Study the drawing (mm; zero at the part's minimum x, y, z) and answer. A direction names the side the tool comes from. Give positions to 0.01 mm unless a question says otherwise; leave off trailing zeros. Write each loop counter-clockwise with the first axis right and the second up, starting at its lowest first coordinate (ties: lowest second). Pieces come first, ordered by that corner, then holes.
1) Find section D-D (y = 28). Determine the outline of the cut face in (x, z).
2) Determine the mould class of the marked faces 4, 5, 6 and 7 for opening direction Y: pulls with the +Y half, pulls with the -Y half, needs draft (parallel to the pull), parting line crosses it, or undercut.
3) Straight lines are drawn through the part: probe 1 along X at (y, z) = (113, 23); probe 2 along Z at (x, y) = (17, 113); probe 3 along Y at (x, z) = (12, 19.5). For each, find the intervals that lie inside material, in ascending order.
4) Find section A-A (z = 23). Determine the outline of the cut face in (x, y).
5) Find section B-B (z = 40). Determine the outline of the cut face in (x, y).
6) Given pin 1 Ø18.5 at (x, z) = (20.5, 32.5) entering from -Y; pin 2 Ø1.2 at (x, z) = (28.5, 2.5) entering from +Y; pin 3 Ø4 at (x, z) = (32, 29) entering from +Y, each flat-ended and moving along its own axis, determine where each tip first touches the part or whether it passes through.
7) Find section C-C (x = 17). Determine the outline of the cut face in (y, z).
8) A tool of negligible diameter and unlimited length cuts with its end or side. For the marked faces 1, 2 and 3, from which of +Z, -Z, +X, -X, +Y, -Y can it reach the whole face along a straight path? Write none if from no direction.
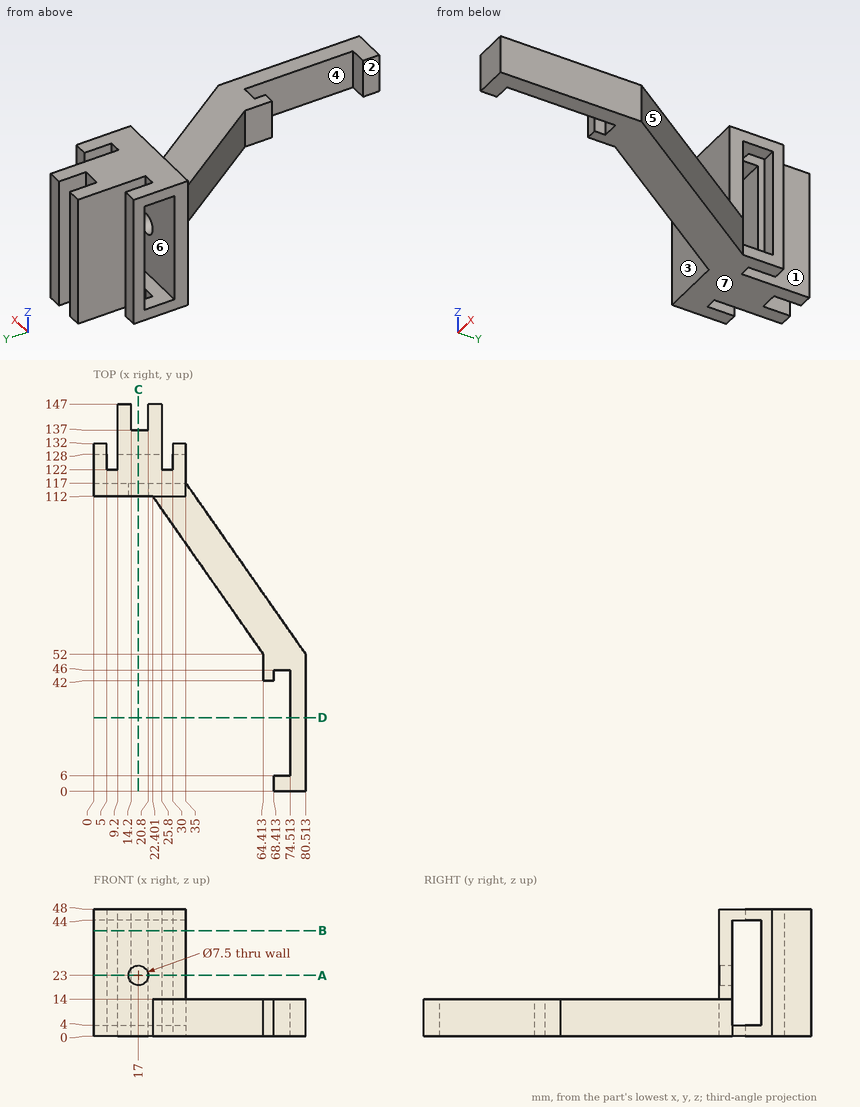
Results:
1. outline: (74.51, 0) - (80.51, 0) - (80.51, 14) - (74.51, 14) - close
2. face 4: undercut
2. face 5: pulls with the +Y half
2. face 6: undercut
2. face 7: needs draft
3. probe 1: x = 0 to 13.25, 20.75 to 35
3. probe 2: z = 0 to 19.25, 26.75 to 48
3. probe 3: y = 112 to 117, 128 to 147
4. outline: (0, 112) - (13.25, 112) - (13.25, 117) - (0, 117) - close; (0, 128) - (5, 128) - (5, 132) - (0, 132) - close; (9.2, 128) - (25.8, 128) - (25.8, 147) - (20.8, 147) - (20.8, 137) - (14.2, 137) - (14.2, 147) - (9.2, 147) - close; (20.75, 112) - (35, 112) - (35, 117) - (20.75, 117) - close; (30, 128) - (35, 128) - (35, 132) - (30, 132) - close
5. outline: (0, 112) - (35, 112) - (35, 117) - (0, 117) - close; (0, 128) - (5, 128) - (5, 132) - (0, 132) - close; (9.2, 128) - (25.8, 128) - (25.8, 147) - (20.8, 147) - (20.8, 137) - (14.2, 137) - (14.2, 147) - (9.2, 147) - close; (30, 128) - (35, 128) - (35, 132) - (30, 132) - close
6. pin 1: stops at y = 112
6. pin 2: stops at y = 122
6. pin 3: stops at y = 132
7. outline: (112, 0) - (137, 0) - (137, 48) - (112, 48) - (112, 26.75) - (117, 26.75) - (117, 44) - (128, 44) - (128, 4) - (117, 4) - (117, 19.25) - (112, 19.25) - close
8. face 1: +Z, -Z, +Y
8. face 2: +Z, -Z, -X, -Y
8. face 3: +Z, -X, -Y
